Build history of the part. All positions in model axes, mm. Coordinates: 2 decimals unless noted, no trailing zeros. Order: outer loops, then holes, each group sorted by start corner. A loop starts at its lowest first (then second) coordinate and runs counter-clockwise, first axis right, second up. Notation, with made-up numbers: (-35, 13.5) - (-4, 13.5) arc R29 cw to (-4, 45.5) - close; hole circle Ø5 at (23.25, 12.5). An arc over 180 degrees is marked (long way). Write each question's results on one line, items separated by ' | '.
from build123d import *

# Parameters (mm, degrees)
SKETCH1_W                        = 12.7
SKETCH1_H                        = 6.0198
BOSS_EXTRUDE1_DEPTH              = 5.7658
SKETCH13_R                       = 0.635
CUT_EXTRUDE2_DEPTH               = 5.7658
CHAMFER1_SIZE                    = 50.8
F_4_CLEARANCE_HOLE1_D            = 2.9464
F_4_CLEARANCE_HOLE1_DEPTH        = 6.35
F_4_CLEARANCE_HOLE1_TIP          = 0.885187864
F_3_8_0_375_DIAMETER_HOLE1_D     = 9.525
F_3_8_0_375_DIAMETER_HOLE1_DEPTH = 6.35
F_3_8_0_375_DIAMETER_HOLE1_TIP   = 2.861598698
CUT_EXTRUDE3_REACH               = 234.708
FILLET3_R                        = 6.35
CUT_EXTRUDE4_REACH               = 234.708
CUT_EXTRUDE5_REACH               = 234.708
SKETCH26_W                       = 2.9591
SKETCH26_H                       = 9.525
CUT_EXTRUDE6_REACH               = 234.708
SKETCH29_W                       = 65.024
SKETCH29_H                       = 36.83
FILLET5_R                        = 6.35
SKETCH30_W                       = 65.151
SKETCH30_H                       = 50.8
BOSS_EXTRUDE2_DEPTH              = 5.7658
FILLET6_R                        = 6.35
CUT_EXTRUDE9_REACH               = 234.708
SKETCH32_W                       = 9.525
SKETCH32_H                       = 2.9591
F_6_CLEARANCE_HOLE1_D            = 3.6576
F_6_CLEARANCE_HOLE1_DEPTH        = 5.842
F_6_CLEARANCE_HOLE1_TIP          = 1.0988539
CUT_EXTRUDE10_REACH              = 234.708
CHAMFER3_SIZE                    = 12.7
CUT_EXTRUDE11_START              = -5.7658
CUT_EXTRUDE11_DEPTH              = 5.7658
CUT_EXTRUDE12_REACH              = 234.708
SKETCH36_W                       = 57.277
SKETCH36_H                       = 36.83
FILLET7_R                        = 2.54
FILLET8_R                        = 6.35
CUT_EXTRUDE13_REACH              = 234.708
SKETCH37_W                       = 9.525
SKETCH37_H                       = 2.9591
F_4_CLEARANCE_HOLE2_D            = 2.9464
F_4_CLEARANCE_HOLE2_DEPTH        = 5.7658
SKETCH38_W                       = 50.8
SKETCH38_H                       = 19.05
CUT_EXTRUDE14_DEPTH              = 233.70795425
FILLET9_R                        = 6.35


with BuildPart() as part:
    # Sketch1 → Boss-Extrude1 (new body)
    with BuildSketch(Plane.XY):
        Polygon((-25.4, 0), (25.4, 0), (25.4, -6.35), (38.1, -6.35), (38.1, 0), (44.45, 0), (44.45, 205.2008), (-109.601, 205.2008), (-109.601, 135.3508), (-44.45, 135.3508), (-44.45, 0), (-38.1, 0), (-38.1, -6.35), (-25.4, -6.35), align=None)
        with Locations((12.7, 9.3599)):
            Rectangle(SKETCH1_W, SKETCH1_H, mode=Mode.SUBTRACT)
        with Locations((-12.7, 9.3599)):
            Rectangle(SKETCH1_W, SKETCH1_H, mode=Mode.SUBTRACT)
    extrude(amount=BOSS_EXTRUDE1_DEPTH)

    # Sketch13 → Cut-Extrude2 (cut)
    with BuildSketch(Plane.XY):
        with Locations((-19.05, 12.3698)):
            Circle(SKETCH13_R)
    cut_extrude2 = extrude(amount=CUT_EXTRUDE2_DEPTH, mode=Mode.SUBTRACT)

    # Sketch-Pattern1: Cut-Extrude2 at 11 more places
    with Locations((12.7, 0, 0), (12.7, -6.0198, 0), (0, -6.0198, 0), (25.4, 0, 0), (38.1, 0, 0), (38.1, -6.0198, 0), (25.4, -6.0198, 0), (57.15, -12.3698, 0), (44.45, -12.3698, 0), (-6.35, -12.3698, 0), (-19.05, -12.3698, 0)):
        add(cut_extrude2, mode=Mode.SUBTRACT)

    # Chamfer1
    chamfer1_edges = [part.edges().sort_by_distance(p)[0] for p in [
        (44.45, 205.2008, 2.8829),
    ]]
    chamfer(chamfer1_edges, length=CHAMFER1_SIZE)

    # #4 Clearance Hole1
    with Locations(Plane.XY.offset(5.7658)):
        with Locations((-31.75, 3.175), (31.75, 3.175), (0, 3.175)):
            Hole(F_4_CLEARANCE_HOLE1_D / 2, depth=F_4_CLEARANCE_HOLE1_DEPTH)
            with Locations((0, 0, -(F_4_CLEARANCE_HOLE1_DEPTH + F_4_CLEARANCE_HOLE1_TIP / 2))):  # 118° drill point
                Cone(0, F_4_CLEARANCE_HOLE1_D / 2, F_4_CLEARANCE_HOLE1_TIP, mode=Mode.SUBTRACT)

    # 3/8 (0.375) Diameter Hole1
    with Locations(Plane.XY.offset(5.7658)):
        with Locations((-100.076, 144.8758), (-100.076, 195.6758)):
            Hole(F_3_8_0_375_DIAMETER_HOLE1_D / 2, depth=F_3_8_0_375_DIAMETER_HOLE1_DEPTH)
            with Locations((0, 0, -(F_3_8_0_375_DIAMETER_HOLE1_DEPTH + F_3_8_0_375_DIAMETER_HOLE1_TIP / 2))):  # 118° drill point
                Cone(0, F_3_8_0_375_DIAMETER_HOLE1_D / 2, F_3_8_0_375_DIAMETER_HOLE1_TIP, mode=Mode.SUBTRACT)

    # Sketch24 → Cut-Extrude3 (cut, up to next)
    with BuildSketch(Plane.XY.offset(5.7658), mode=Mode.PRIVATE) as cut_extrude3_sk1:
        Polygon((31.75, 167.1008), (31.75, 16.002), (44.45, 16.002), (44.45, 154.4008), align=None)
    cut_extrude3_tool1 = extrude(cut_extrude3_sk1.sketch, amount=-CUT_EXTRUDE3_REACH, mode=Mode.PRIVATE) & part.part
    add(cut_extrude3_tool1.solids().sort_by_distance((38.007144, 88.422828, 5.7658))[0], mode=Mode.SUBTRACT)

    # Fillet3
    fillet3_edges = [part.edges().sort_by_distance(p)[0] for p in [
        (31.75, 16.002, 2.8829),
    ]]
    fillet(fillet3_edges, radius=FILLET3_R)

    # Sketch25 → Cut-Extrude4 (cut, up to next)
    with BuildSketch(Plane.XY.offset(5.7658), mode=Mode.PRIVATE) as cut_extrude4_sk1:
        with BuildLine():
            ThreePointArc((-20.441531288, 134.8428), (-19.812, 144.8758), (-20.441531288, 154.9088))
            ThreePointArc((-20.441531288, 154.9088), (-24.981656286, 158.432924998), (-28.505781284, 153.8928))
            ThreePointArc((-28.505781284, 153.8928), (-27.94, 144.8758), (-28.505781284, 135.8588))
            ThreePointArc((-28.505781284, 135.8588), (-24.981656286, 131.318675002), (-20.441531288, 134.8428))
        make_face()
    cut_extrude4_tool1 = extrude(cut_extrude4_sk1.sketch, amount=-CUT_EXTRUDE4_REACH, mode=Mode.PRIVATE) & part.part
    # Sketch25 → Cut-Extrude4 (cut, up to next)
    with BuildSketch(Plane.XY.offset(5.7658), mode=Mode.PRIVATE) as cut_extrude4_sk2:
        with BuildLine():
            ThreePointArc((17.359640569, 130.0803), (18.288, 144.8758), (17.359640569, 159.6713))
            ThreePointArc((17.359640569, 159.6713), (12.819515571, 163.195424998), (9.295390572, 158.6553))
            ThreePointArc((9.295390572, 158.6553), (10.16, 144.8758), (9.295390572, 131.0963))
            ThreePointArc((9.295390572, 131.0963), (12.819515571, 126.556175002), (17.359640569, 130.0803))
        make_face()
    cut_extrude4_tool2 = extrude(cut_extrude4_sk2.sketch, amount=-CUT_EXTRUDE4_REACH, mode=Mode.PRIVATE) & part.part
    add(cut_extrude4_tool1.solids().sort_by_distance((-24.175106, 144.8758, 5.7658))[0], mode=Mode.SUBTRACT)
    add(cut_extrude4_tool2.solids().sort_by_distance((13.816141, 144.8758, 5.7658))[0], mode=Mode.SUBTRACT)

    # Sketch26 → Cut-Extrude5 (cut, up to next)
    with BuildSketch(Plane.XY.offset(5.7658), mode=Mode.PRIVATE) as cut_extrude5_sk1:
        with Locations((9.35355, 61.214)):
            Rectangle(SKETCH26_W, SKETCH26_H)
    cut_extrude5_tool1 = extrude(cut_extrude5_sk1.sketch, amount=-CUT_EXTRUDE5_REACH, mode=Mode.PRIVATE) & part.part
    # Sketch26 → Cut-Extrude5 (cut, up to next)
    with BuildSketch(Plane.XY.offset(5.7658), mode=Mode.PRIVATE) as cut_extrude5_sk2:
        with Locations((-19.00555, 61.214)):
            Rectangle(SKETCH26_W, SKETCH26_H)
    cut_extrude5_tool2 = extrude(cut_extrude5_sk2.sketch, amount=-CUT_EXTRUDE5_REACH, mode=Mode.PRIVATE) & part.part
    add(cut_extrude5_tool1.solids().sort_by_distance((9.35355, 61.214, 5.7658))[0], mode=Mode.SUBTRACT)
    add(cut_extrude5_tool2.solids().sort_by_distance((-19.00555, 61.214, 5.7658))[0], mode=Mode.SUBTRACT)

    # Sketch29 → Cut-Extrude6 (cut, up to next)
    with BuildSketch(Plane.XY.offset(5.7658), mode=Mode.PRIVATE) as cut_extrude6_sk1:
        with Locations((-0.762, 186.7858)):
            Rectangle(SKETCH29_W, SKETCH29_H)
    cut_extrude6_tool1 = extrude(cut_extrude6_sk1.sketch, amount=-CUT_EXTRUDE6_REACH, mode=Mode.PRIVATE) & part.part
    add(cut_extrude6_tool1.solids().sort_by_distance((-0.762, 186.7858, 5.7658))[0], mode=Mode.SUBTRACT)

    # Fillet5
    fillet5_edges = [part.edges().sort_by_distance(p)[0] for p in [
        (-33.274, 168.3708, 2.8829),
    ]]
    fillet(fillet5_edges, radius=FILLET5_R)

    # Sketch30 → Boss-Extrude2 (add)
    with BuildSketch(Plane.XY.offset(5.7658)):
        with Locations((-77.0255, 109.9508)):
            Rectangle(SKETCH30_W, SKETCH30_H)
    extrude(amount=-BOSS_EXTRUDE2_DEPTH)

    # Fillet6
    fillet6_edges = [part.edges().sort_by_distance(p)[0] for p in [
        (-44.45, 84.5508, 2.8829),
    ]]
    fillet(fillet6_edges, radius=FILLET6_R)

    # Sketch32 → Cut-Extrude9 (cut, up to next)
    with BuildSketch(Plane.XY.offset(5.7658), mode=Mode.PRIVATE) as cut_extrude9_sk1:
        with Locations((20.6375, 166.0975)):
            Rectangle(SKETCH32_W, SKETCH32_H)
    cut_extrude9_tool1 = extrude(cut_extrude9_sk1.sketch, amount=-CUT_EXTRUDE9_REACH, mode=Mode.PRIVATE) & part.part
    add(cut_extrude9_tool1.solids().sort_by_distance((20.6375, 166.0975, 5.7658))[0], mode=Mode.SUBTRACT)

    # #6 Clearance Hole1
    with Locations(Plane.XY.offset(5.7658)):
        with Locations((-97.0255, 117.65), (-57.0255, 117.65), (-97.0255, 92.65), (-57.0255, 92.65)):
            Hole(F_6_CLEARANCE_HOLE1_D / 2, depth=F_6_CLEARANCE_HOLE1_DEPTH)
            with Locations((0, 0, -(F_6_CLEARANCE_HOLE1_DEPTH + F_6_CLEARANCE_HOLE1_TIP / 2))):  # 118° drill point
                Cone(0, F_6_CLEARANCE_HOLE1_D / 2, F_6_CLEARANCE_HOLE1_TIP, mode=Mode.SUBTRACT)

    # Sketch31 → Cut-Extrude10 (cut, up to next)
    with BuildSketch(Plane.XY.offset(5.7658), mode=Mode.PRIVATE) as cut_extrude10_sk1:
        with BuildLine():
            Line((-12.446, 77.0763), (-12.446, 115.1763))
            ThreePointArc((-12.446, 115.1763), (-4.826, 122.7963), (2.794, 115.1763))
            Line((2.794, 115.1763), (2.794, 77.0763))
            ThreePointArc((2.794, 77.0763), (-4.826, 69.4563), (-12.446, 77.0763))
        make_face()
    cut_extrude10_tool1 = extrude(cut_extrude10_sk1.sketch, amount=-CUT_EXTRUDE10_REACH, mode=Mode.PRIVATE) & part.part
    add(cut_extrude10_tool1.solids().sort_by_distance((-4.826, 96.1263, 5.7658))[0], mode=Mode.SUBTRACT)

    # Chamfer3
    chamfer3_edges = [part.edges().sort_by_distance(p)[0] for p in [
        (-109.601, 84.5508, 2.8829),
    ]]
    chamfer(chamfer3_edges, length=CHAMFER3_SIZE)

    # Sketch35 → Cut-Extrude11 (cut)
    with BuildSketch(Plane.XY.offset(5.7658).offset(CUT_EXTRUDE11_START)):
        Polygon((31.75, 63.5), (15.875, 63.5), (15.875, 126.5243), (9.263515571, 126.5243), (9.263515571, 168.3708), (31.75, 168.3708), align=None)
    extrude(amount=CUT_EXTRUDE11_DEPTH, mode=Mode.SUBTRACT)

    # Sketch36 → Cut-Extrude12 (cut, up to next)
    with BuildSketch(Plane.XY.offset(5.7658), mode=Mode.PRIVATE) as cut_extrude12_sk1:
        with Locations((-55.5625, 186.7858)):
            Rectangle(SKETCH36_W, SKETCH36_H)
    cut_extrude12_tool1 = extrude(cut_extrude12_sk1.sketch, amount=-CUT_EXTRUDE12_REACH, mode=Mode.PRIVATE) & part.part
    add(cut_extrude12_tool1.solids().sort_by_distance((-55.5625, 186.7858, 5.7658))[0], mode=Mode.SUBTRACT)

    # Fillet7
    fillet7_edges = [part.edges().sort_by_distance(p)[0] for p in [
        (15.875, 63.5, 2.8829),
        (9.263515571, 126.5243, 2.8829),
    ]]
    fillet(fillet7_edges, radius=FILLET7_R)

    # Fillet8
    fillet8_edges = [part.edges().sort_by_distance(p)[0] for p in [
        (-84.201, 168.3708, 2.8829),
    ]]
    fillet(fillet8_edges, radius=FILLET8_R)

    # Sketch37 → Cut-Extrude13 (cut, up to next)
    with BuildSketch(Plane.XY.offset(5.7658), mode=Mode.PRIVATE) as cut_extrude13_sk1:
        with Locations((-46.298984429, 165.30375)):
            Rectangle(SKETCH37_W, SKETCH37_H)
    cut_extrude13_tool1 = extrude(cut_extrude13_sk1.sketch, amount=-CUT_EXTRUDE13_REACH, mode=Mode.PRIVATE) & part.part
    add(cut_extrude13_tool1.solids().sort_by_distance((-46.298984, 165.30375, 5.7658))[0], mode=Mode.SUBTRACT)

    # #4 Clearance Hole2
    with Locations(Plane.XY.offset(5.7658)):
        with Locations((-24.1681, 61.214), (14.5161, 61.214), (20.6375, 117.5708), (-100.076, 182.9758), (-100.076, 157.5758), (-62.173984429, 165.30375), (-30.423984429, 165.30375)):
            Hole(F_4_CLEARANCE_HOLE2_D / 2, depth=F_4_CLEARANCE_HOLE2_DEPTH)

    # Sketch38 → Cut-Extrude14 (cut, through all)
    with BuildSketch(Plane.XY.offset(5.7658)):
        with Locations((-6.35, 34.5948)):
            Rectangle(SKETCH38_W, SKETCH38_H)
    extrude(amount=-CUT_EXTRUDE14_DEPTH, mode=Mode.SUBTRACT)

    # Fillet9
    fillet9_edges = [part.edges().sort_by_distance(p)[0] for p in [
        (19.05, 44.1198, 2.8829),
        (19.05, 25.0698, 2.8829),
        (-31.75, 25.0698, 2.8829),
        (-31.75, 44.1198, 2.8829),
    ]]
    fillet(fillet9_edges, radius=FILLET9_R)


solid = part.part
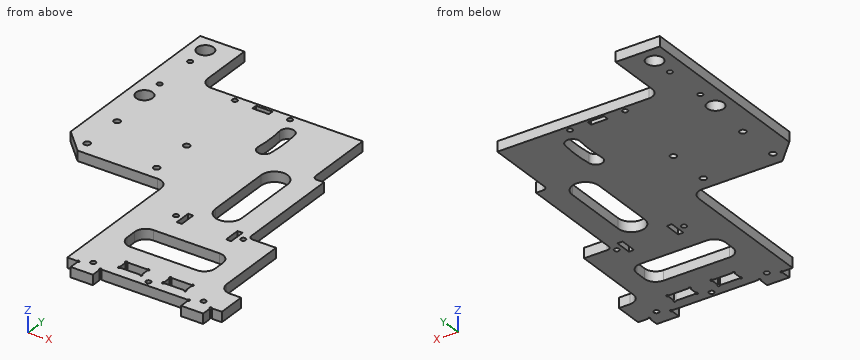
1. Drop flat-ended pins along their axis: pin 1 Ø2 at (x, y) = (-12, 129) entering from -Z; pin 2 Ø1.7 at (y, z) = (61, 1.5) entering from +X; pin 3 Ø3 at (y, z) = (35.5, 2.5) entering from +X; pin 4 Ø2.5 at (x, z) = (-19.5, 1.5) entering from -Y. Give the stop position or say it passes through.
Solved:
pin 1: stops at z = 0 | pin 2: stops at x = 31.75 | pin 3: stops at x = 31.75 | pin 4: stops at y = 0
2. Probe line 1 (X direction, y = 58, z = 5); line 2 (X direction, y = 6.5, z = 4.25); line 3 (Y direction, x = -44, z = 3.05). List the from-to ranges inside material, lowest first.
Solved:
line 1: x = -44.45 to -20.49, -17.53 to 7.87, 10.83 to 31.75 | line 2: x = -44.45 to -19.67, -5.73 to 5.73, 19.67 to 44.45 | line 3: y = 0 to 163.82, 166.78 to 168.37
3. Band-saw the part on B-B on z = 3.4. Give the number of separate pieces and of enclosed holes in the cut face, then the cut area to 3 significant figures.
Solved:
separate pieces: 1 | enclosed holes: 23 | area: 15,200 mm2
4. Band-saw the part on A-A on y = 108. Give the cut face in (x, z) (3 decimals).
Solved:
outline: (-109.601, 0) - (-12.446, 0) - (-12.446, 5.766) - (-109.601, 5.766) - close; (2.794, 0) - (15.875, 0) - (15.875, 5.766) - (2.794, 5.766) - close
